Can you work these out from the model? Positions are in its coordinate system, mm. A direction names the side the tool comes from. Round coordinates to 2 decimals unless told otherwise and drop trailing zeros. Write each loop counter-clockwise with the first axis right and the second up, starting at its lowest first coordinate (ties: lowest second). Pieces come first, ordered by that corner, then holes.
Q1. For faces 4 (the flat face through (12, 25, 29)), 5 (the flat face through (21.277, 25, 25)), 6 (the flat face through (10, 38.286, 26)), 7 (the flat face through (12, 26, -25)), which set-ups out of +Z, -Z, +X, -X, +Y, -Y let a thin tool reach every point of the face, with its end or its side?
Q2. I'm going to push flat-ended pins straight in: pin 1 Ø15.5 at (x, y) = (9.5, 28.5) entering from -Z; pin 2 Ø8 at (y, z) = (40.5, -22) entering from +X; pin 3 Ø3 at (x, z) = (12, 25.5) entering from +Y. Where does each tip first touch, or does it pass through?
Q3. We'd pull the mould along Z, two halves only. Please class faces 1 (the flat face through (8.848, 40, -25)), 2 (the cylindrical face through (-28.797, 2.465, 28.859)), 3 (the flat face through (11, 25, 22)): +Z half, -Z half, draft (parallel to the pull), parting line (faces both ways), or undercut.
Q4. If we section it at B-B (y = 31): Please give me the cut outline in (x, z), plus the area to 3 significant figures.
Q5. If we section it at D-D (x = 12): Give the number of separate pieces and of enclosed holes in the cut face, plus the area to 3 significant figures.
Q6. If we section it at C-C (z = 11): Please give me the cut outline in (x, y), plus the area to 3 significant figures.
Q7. Please list where these lines run through material, in increasing order: line 1 along Z through (x, y) = (12, 33.75); line 2 along Z through (x, y) = (-25, 1.95); line 3 along Z through (x, y) = (3, 43).
Q8. If we section it at A-A (x = -25): Please give me the cut outline in (y, z).
Autodesk Inventor part; units mm, degrees
ref_plane "YZ Plane" through (0, 0, 0) normal (1, 0, 0) x (0, 1, 0)
ref_plane "XZ Plane" through (0, 0, 0) normal (0, 1, 0) x (-1, 0, 0)
ref_plane "XY Plane" through (0, 0, 0) normal (0, 0, 1) x (1, 0, 0)
sketch "Szkic1" plane through (0, 0, 0) normal (0, 1, 0) x (-1, 0, 0)
  line L0 (-26, 30) -> (26, 30)
  line L1 (30, 26) -> (30, -26)
  line L2 (26, -30) -> (-26, -30)
  line L3 (-30, -26) -> (-30, 26)
  line L4 (-30, 30) -> (30, -30) construction
  line L5 (30, 30) -> (-30, -30) construction
  circle A0 centre (-25, -25) radius 1.5
  circle A1 centre (25, 11) radius 1.5
  arc A2 (-30, -26) -> (-26, -30) centre (-26, -26) ccw
  arc A3 (-26, 30) -> (-30, 26) centre (-26, 26) ccw
  arc A4 (30, 26) -> (26, 30) centre (26, 26) ccw
  arc A5 (26, -30) -> (30, -26) centre (26, -26) ccw
  point P0 (0, 0)
  dimension "d0" = 60
  dimension "d1" = 60
  dimension "d2" = 3
  dimension "d3" = 3
  dimension "d5" = 4
  dimension "d6" = 4
  dimension "d7" = 4
  dimension "d8" = 4
extrude "Wyciągnięcie proste1" add sketch "Szkic1" along normal blind 5
sketch "Szkic2" plane through (0, 5, 0) normal (0, 1, 0) x (1, 0, 0)
  line L0 (21.8475, 21.1097) -> (1.8475, 21.1097)
  line L1 (1.8475, 21.1097) -> (1.8475, 28.1097)
  line L2 (1.8475, 28.1097) -> (21.8475, 28.1097)
  line L3 (21.8475, 28.1097) -> (21.8475, 21.1097)
  line L4 (1.8475, -22) -> (21.2771, -22)
  line L5 (21.2771, -22) -> (21.2771, -29)
  line L6 (21.2771, -29) -> (1.8475, -29)
  line L7 (1.8475, -29) -> (1.8475, -22)
  point P0 (0, 0)
  dimension "d11" = 20
  dimension "d12" = 7
  dimension "d13" = 7
extrude "Wyciągnięcie proste2" add sketch "Szkic2" along normal blind 41
sketch "Szkic3" plane through (1.8475, 5, 29) normal (0, 0, 1) x (1, 0, 0)
  line L0 (7, 33.2857) -> (13, 33.2857)
  line L1 (13, 33.2857) -> (13, 36.7143)
  line L2 (13, 36.7143) -> (7, 36.7143)
  line L3 (7, 36.7143) -> (7, 33.2857)
  line L4 (7, 33.2857) -> (13, 36.7143) construction
  line L5 (13, 33.2857) -> (7, 36.7143) construction
  point P0 (-1.8475, -5)
  point P1 (10, 35)
  dimension "d16" = 6
  dimension "d17" = 3.4286
sketch "Szkic4" plane through (1.8475, 5, -21.1097) normal (0, 0, 1) x (1, 0, 0)
  line L0 (7, 33.2857) -> (13, 33.2857)
  line L1 (13, 33.2857) -> (13, 36.7143)
  line L2 (13, 36.7143) -> (7, 36.7143)
  line L3 (7, 36.7143) -> (7, 33.2857)
  line L4 (7, 33.2857) -> (13, 36.7143) construction
  line L5 (13, 33.2857) -> (7, 36.7143) construction
  point P0 (-1.8475, -5)
  point P1 (10, 35)
  dimension "d18" = 6
  dimension "d19" = 3.4286
extrude "Wyciągnięcie proste3" cut sketch "Szkic4" against normal blind 7
extrude "Wyciągnięcie proste4" cut sketch "Szkic3" against normal blind 7
sketch "Szkic5" plane through (0, 46, 0) normal (0, 1, 0) x (1, 0, 0)
  circle A0 centre (12, 24.5) radius 1.75
  circle A1 centre (12, -25.5) radius 1.75
  point P0 (0, 0)
  dimension "d24" = 3.5
  dimension "d25" = 3.5
extrude "Wyciągnięcie proste5" cut sketch "Szkic5" against normal blind 20
properties part number "MotorHolder"
A:
1. face 4: +Z, +X, -X, +Y
1. face 5: +Z, +X, +Y
1. face 6: +Z, -Z
1. face 7: +Y
2. pin 1: stops at z = -28.11
2. pin 2: stops at x = 21.85
2. pin 3: stops at y = 26
3. face 1: draft
3. face 2: +Z half
3. face 3: undercut
4. outline: (1.85, -28.11) - (21.85, -28.11) - (21.85, -21.11) - (1.85, -21.11) - close; (1.85, 22) - (21.28, 22) - (21.28, 29) - (1.85, 29) - close; hole circle Ø3.5 at (12, -24.5); hole circle Ø3.5 at (12, 25.5)
4. area: 257 mm2
5. separate pieces: 5
5. enclosed holes: 0
5. area: 710 mm2
6. outline: (-30, 0) - (-26.5, 0) - (-26.5, 5) - (-30, 5) - close; (-23.5, 0) - (30, 0) - (30, 5) - (-23.5, 5) - close
6. area: 285 mm2
7. line 1: z = -28.11 to -26.25, -22.75 to -21.11, 22 to 23.75, 27.25 to 29
7. line 2: z = -30 to 9.5, 12.5 to 30
7. line 3: z = -28.11 to -21.11, 22 to 29
8. outline: (0, -30) - (5, -30) - (5, 9.5) - (0, 9.5) - close; (0, 12.5) - (5, 12.5) - (5, 30) - (0, 30) - close
